Verification items for this drawing (mm, ordinates from the low corner). Round coordinates to 2 decimals unless told otherwise and drop trailing zeros. Order: outer loops, then holes, each group sorted by start corner. A loop starts at its lowest first (then second) coordinate and runs counter-clockwise, first axis right, second up. Notation, with made-up numbers: (67.5, 66) - (84.5, 66) arc R18 ccw to (84.5, 83) - close; hole circle Ø6 at (27, 43). An arc over 180 degrees is marked (long way). Return JSON: item names as keys, results as strings. Group by question number.
Q1. Material ranges on line 1 along Z through (x, y) = (1.45, 1.8); line 2 along X through (y, z) = (2.5, 1.5); line 3 along Y through (x, z) = (1.3, 15.5), recorded low to high.
Q2. Sectioned sample at A-A, the plane z = 7.5. Record the cut outline in (x, y) (3 decimals), then the cut area to 4 significant figures.
Q3. Draft check along Y on the marked faces 1 and 2. Enter one of: pulls with the +Y half, pulls with the -Y half, needs draft (parallel to the pull), parting line crosses it, or undercut.
Q4. Gauge pin test, flat ends, axial feed: pin 1 Ø2.5 at (x, y) = (2.775, 2.775) entering from -Z; pin 2 Ø2 at (y, z) = (4.5, 8) entering from -X; pin 3 Ø1 at (y, z) = (0.5, 7.5) entering from +X. Record the tip position at first contact, or that the pin passes through.
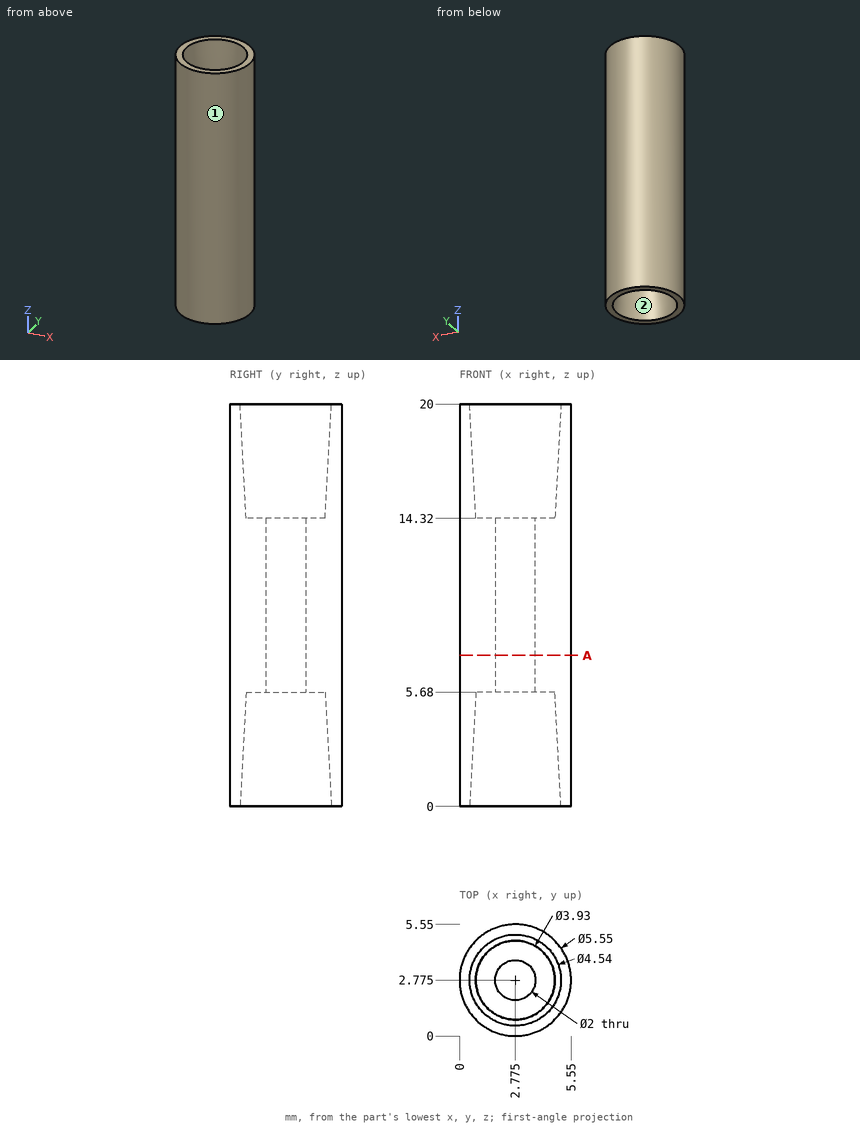
Reply:
{
 "1": {"line 1": "5.68 to 14.32", "line 2": "0.01 to 0.6, 4.95 to 5.54", "line 3": "0.42 to 1.38, 4.17 to 5.13"},
 "2": {"outline": "circle Ø5.55 at (2.775, 2.775); hole circle Ø2 at (2.775, 2.775)", "area": "21.05 mm^2"},
 "3": {"face 1": "parting line crosses it", "face 2": "undercut"},
 "4": {"pin 1": "z = 5.68", "pin 2": "x = 0.1", "pin 3": "x = 4.91"}
}
